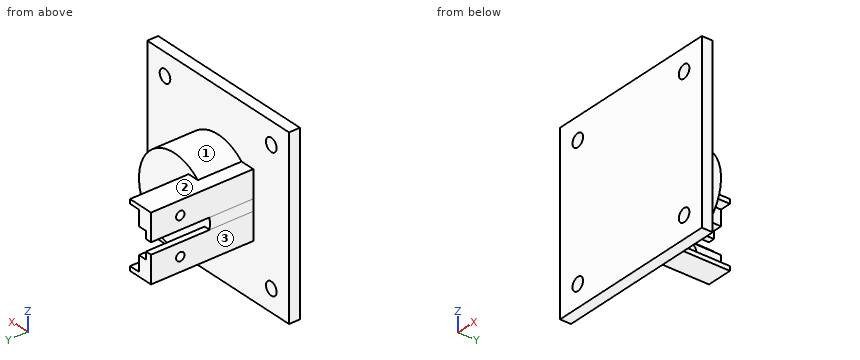
```python
from build123d import *

# Parameters (mm, degrees)
SKETCH1_R                 = 12.7
BOSS_EXTRUDE1_DEPTH       = 12.7
BOSS_EXTRUDE2_DEPTH       = 17
CUT_EXTRUDE3_DEPTH        = 17
BOSS_EXTRUDE4_REACH       = 36.708
F_2_CLEARANCE_HOLE1_D     = 2.4384
F_2_CLEARANCE_HOLE1_DEPTH = 25.4
F_2_CLEARANCE_HOLE1_TIP   = 0.732569267
SKETCH14_W                = 50.8
SKETCH14_H                = 50.8
BOSS_EXTRUDE7_DEPTH       = 3.175
F_6_CLEARANCE_HOLE1_D     = 3.7973
F_6_CLEARANCE_HOLE1_DEPTH = 25.4
F_6_CLEARANCE_HOLE1_TIP   = 1.140824014


with BuildPart() as part:
    # Sketch1 → Boss-Extrude1 (new body)
    with BuildSketch(Plane(origin=(0, 0, 0), x_dir=(1, 0, 0), z_dir=(0, 1, 0))):
        with Locations(Location((0, 0, 0), (0, 0, 270))):
            Circle(SKETCH1_R)
    extrude(amount=BOSS_EXTRUDE1_DEPTH)

    # Sketch7 → Boss-Extrude2 (add)
    with BuildSketch(Plane(origin=(0, 12.7, 0), x_dir=(1, 0, 0), z_dir=(0, 1, 0))):
        with BuildLine():
            ThreePointArc((-8.400260413, 9.525), (-11.575260413, 5.225260413), (-12.7, 0))
            ThreePointArc((-12.7, 0), (-11.575260413, -5.225260413), (-8.400260413, -9.525))
            Line((-8.400260413, -9.525), (-5.08, -9.525))
            Line((-5.08, -9.525), (-5.08, -8.255))
            Line((-5.08, -8.255), (-8.255, -8.255))
            Line((-8.255, -8.255), (-8.255, 8.255))
            Line((-8.255, 8.255), (-5.08, 8.255))
            Line((-5.08, 8.255), (-5.08, 9.525))
            Line((-5.08, 9.525), (-8.400260413, 9.525))
        make_face()
    extrude(amount=BOSS_EXTRUDE2_DEPTH)

    # Sketch8 → Cut-Extrude3 (cut)
    with BuildSketch(Plane(origin=(0, 29.7, 0), x_dir=(1, 0, 0), z_dir=(0, 1, 0))):
        Polygon((-8.255, -3.81), (-8.255, 3.81), (-10.795, 3.81), (-10.795, 1.651), (-12.7, 1.651), (-12.7, -1.651), (-10.795, -1.651), (-10.795, -3.81), align=None)
    extrude(amount=-CUT_EXTRUDE3_DEPTH, mode=Mode.SUBTRACT)

    # Boss-Extrude4: up to this face of the body (flat: up to its plane)
    boss_extrude4_end = Plane(part.part.faces().sort_by_distance((0, 0, 0))[0])
    # Sketch13 → Boss-Extrude4 (add, up to the picked face)
    with BuildSketch(Plane(origin=(0, 29.7, 0), x_dir=(1, 0, 0), z_dir=(0, 1, 0)), mode=Mode.PRIVATE) as boss_extrude4_sk1:
        with BuildLine():
            Line((-12.592227722, 1.651), (-12.592227722, 9.525))
            Line((-12.592227722, 9.525), (-8.400260413, 9.525))
            ThreePointArc((-8.400260413, 9.525), (-11.210312597, 5.968156456), (-12.592227722, 1.651))
        make_face()
    boss_extrude4_tool1 = split(extrude(boss_extrude4_sk1.sketch, amount=-BOSS_EXTRUDE4_REACH, mode=Mode.PRIVATE), bisect_by=boss_extrude4_end, keep=Keep.BOTH, mode=Mode.PRIVATE)
    # Sketch13 → Boss-Extrude4 (add, up to the picked face)
    with BuildSketch(Plane(origin=(0, 29.7, 0), x_dir=(1, 0, 0), z_dir=(0, 1, 0)), mode=Mode.PRIVATE) as boss_extrude4_sk2:
        with BuildLine():
            Line((-12.592227722, -1.651), (-12.592227722, -9.525))
            Line((-12.592227722, -9.525), (-8.400260413, -9.525))
            ThreePointArc((-8.400260413, -9.525), (-11.210312597, -5.968156456), (-12.592227722, -1.651))
        make_face()
    boss_extrude4_tool2 = split(extrude(boss_extrude4_sk2.sketch, amount=-BOSS_EXTRUDE4_REACH, mode=Mode.PRIVATE), bisect_by=boss_extrude4_end, keep=Keep.BOTH, mode=Mode.PRIVATE)
    add(boss_extrude4_tool1.solids().sort_by(Axis((-11.366083, 29.7, -7.381946), (0, -1, 0)))[0])
    add(boss_extrude4_tool2.solids().sort_by(Axis((-11.366083, 29.7, 7.381946), (0, -1, 0)))[0])

    # #2 Clearance Hole1
    with Locations(Plane(origin=(-8.255, 0, 0), x_dir=(0, 0, -1), z_dir=(1, 0, 0))):
        with Locations((-5.46, 21.2), (5.46, 21.2)):
            Hole(F_2_CLEARANCE_HOLE1_D / 2, depth=F_2_CLEARANCE_HOLE1_DEPTH)
            with Locations((0, 0, -(F_2_CLEARANCE_HOLE1_DEPTH + F_2_CLEARANCE_HOLE1_TIP / 2))):  # 118° drill point
                Cone(0, F_2_CLEARANCE_HOLE1_D / 2, F_2_CLEARANCE_HOLE1_TIP, mode=Mode.SUBTRACT)

    # Sketch14 → Boss-Extrude7 (add)
    with BuildSketch(Plane.XZ):
        Rectangle(SKETCH14_W, SKETCH14_H)
    extrude(amount=BOSS_EXTRUDE7_DEPTH)

    # #6 Clearance Hole1
    with Locations(Plane(origin=(0, -3.175, 0), x_dir=(-1, 0, 0), z_dir=(0, -1, 0))):
        with Locations((19.05, -19.05), (-19.05, -19.05), (-19.05, 19.05), (19.05, 19.05)):
            Hole(F_6_CLEARANCE_HOLE1_D / 2, depth=F_6_CLEARANCE_HOLE1_DEPTH)
            with Locations((0, 0, -(F_6_CLEARANCE_HOLE1_DEPTH + F_6_CLEARANCE_HOLE1_TIP / 2))):  # 118° drill point
                Cone(0, F_6_CLEARANCE_HOLE1_D / 2, F_6_CLEARANCE_HOLE1_TIP, mode=Mode.SUBTRACT)


solid = part.part
```
Here's how the part is built. I have some questions about the finished solid (model axes, mm). Face numbers are marked on the shaded views. A direction names the side the tool comes from. Give positions to 0.01 mm unless a question says otherwise; leave off trailing zeros. Write each loop counter-clockwise with the first axis right and the second up, starting at its lowest first coordinate (ties: lowest second). Pieces come first, ordered by that corner, then holes. Notation, with made-up numbers: (84, -33) -> (123, -33) arc R18 cw to (123, -11) -> close; hole circle Ø4 at (46.5, 46). An arc over 180 degrees is marked (long way). Write each question's results on one line, items separated by ' | '.
Item 1: On a 3-axis mill with a long thin cutter (end or side, diameter ignored), from which of +Z, -Z, +X, -X, +Y, -Y can I reach the whole of each face in a straight line? I mean the marked faces 1, 2 and 3. Say none if no direction works.
Output:
face 1: +Y | face 2: +Z, -X, +Y | face 3: -Z, -X, +Y
Item 2: For pin 1 Ø2.5 at (x, y) = (-9.5, 21.5) entering from +Z (3 decimals); pin 2 Ø1.4 at (y, z) = (25, 9) entering from +X; pin 3 Ø3 at (x, z) = (-10, -16.5) entering from +Y, each with a flat end and sliding along its axis, tell me the tip position at first contact or that it passes through.
Output:
pin 1: stops at z = 9.525 | pin 2: stops at x = -5.08 | pin 3: stops at y = 0
Item 3: Suppose I cut it at C-C on x = 19.05. Write out the boundary of the cut face in (y, z) (3 decimals).
Output:
outline: (-3.175, -25.4) -> (0, -25.4) -> (0, -20.949) -> (-3.175, -20.949) -> close; (-3.175, -17.151) -> (0, -17.151) -> (0, 17.151) -> (-3.175, 17.151) -> close; (-3.175, 20.949) -> (0, 20.949) -> (0, 25.4) -> (-3.175, 25.4) -> close
Item 4: Suppose I cut it at A-A on y = -1. Write out the boundary of the cut face in (x, z), plus the area to 3 significant figures.
Output:
outline: (-25.4, -25.4) -> (25.4, -25.4) -> (25.4, 25.4) -> (-25.4, 25.4) -> close; hole circle Ø3.8 at (-19.05, -19.05); hole circle Ø3.8 at (-19.05, 19.05); hole circle Ø3.8 at (19.05, -19.05); hole circle Ø3.8 at (19.05, 19.05) | area: 2,540 mm^2
Item 5: Suppose I cut it at D-D on y = 21.2. Write out the boundary of the cut face in (x, z) (3 decimals).
Output:
outline: (-12.592, -9.525) -> (-5.08, -9.525) -> (-5.08, -8.255) -> (-8.255, -8.255) -> (-8.255, -6.679) -> (-12.592, -6.679) -> close; (-12.592, -4.241) -> (-8.255, -4.241) -> (-8.255, -3.81) -> (-10.795, -3.81) -> (-10.795, -1.651) -> (-12.592, -1.651) -> close; (-12.592, 1.651) -> (-10.795, 1.651) -> (-10.795, 3.81) -> (-8.255, 3.81) -> (-8.255, 4.241) -> (-12.592, 4.241) -> close; (-12.592, 6.679) -> (-8.255, 6.679) -> (-8.255, 8.255) -> (-5.08, 8.255) -> (-5.08, 9.525) -> (-12.592, 9.525) -> close
Item 6: Suppose I cut it at B-B on z = -19.05. Write out the boundary of the cut face in (x, y) (3 decimals).
Output:
outline: (-25.4, -3.175) -> (-20.949, -3.175) -> (-20.949, 0) -> (-25.4, 0) -> close; (-17.151, -3.175) -> (17.151, -3.175) -> (17.151, 0) -> (-17.151, 0) -> close; (20.949, -3.175) -> (25.4, -3.175) -> (25.4, 0) -> (20.949, 0) -> close
Item 7: If I drill on L1, parallel to X at y = -2, z = 19.05; L2, parallel to Y at x = -3.5, z = 22 (3 decimals), over which ranges is the centre line in solid material (lowest first)?
Output:
L1: x = -25.4 to -20.95, -17.15 to 17.15, 20.95 to 25.4 | L2: y = -3.175 to 0
